```python
from build123d import *

# Parameters (mm, degrees)
BOSS_EXTRUDE2_DEPTH     = 8.3
CIRPATTERN1_COUNT       = 4
SKETCH13_R              = 22.4
CUT_EXTRUDE3_DEPTH      = 4
FILLET1_R               = 5
SKETCH15_R              = 18
SKETCH15_R_2            = 15
BOSS_EXTRUDE3_DEPTH     = 4
SKETCH16_R              = 7.5
CUT_EXTRUDE4_DEPTH      = 103.587698187
FILLET2_R               = 5
FILLET4_R               = 3
FILLET5_R               = 2
FILLET6_R               = 2
TAP_DRILL_FOR_M6_TAP1_D = 5
CIRPATTERN2_COUNT       = 4


with BuildPart() as part:
    # Sketch1 → Revolve1 (revolve)
    with BuildSketch(Plane.XY, mode=Mode.PRIVATE) as revolve1_sk:
        Polygon((22.3, -26.9), (53.8, -26.9), (53.8, 0.95810827), (56.6, 0.95810827), (56.6, 3.75810827), (59, 3.75810827), (59, 0), (59, -31.9), (0, -31.9), (0, -26.9), (17.5, -26.9), (17.5, -6.8), (22.3, -6.8), align=None)
    revolve(revolve1_sk.sketch.rotate(Axis((0, -26.9, 0), (0, -1, 0)), 180), axis=Axis((0, -26.9, 0), (0, -1, 0)))

    # Sketch2 → Boss-Extrude2 (add)
    with BuildSketch(Plane(origin=(0, 3.75810827, 0), x_dir=(1, 0, 0), z_dir=(0, 1, 0))):
        Polygon((7.756499668, 69), (-8.243500332, 69), (-11.893500332, 57.788793462), (11.406499668, 57.88688768), align=None)
    boss_extrude2 = extrude(amount=-BOSS_EXTRUDE2_DEPTH)

    # CirPattern1: Boss-Extrude2 ×4 about axis
    cirpattern1_axis = Axis((0, 0, 0), (0, 1, 0))
    for i in range(1, CIRPATTERN1_COUNT):
        add(boss_extrude2.rotate(cirpattern1_axis, i * 360 / CIRPATTERN1_COUNT))

    # Sketch10 → Cut-Revolve4 (revolve, cut)
    with BuildSketch(Plane(origin=(0, 0, 0), x_dir=(0, 0, -1), z_dir=(1, 0, 0)), mode=Mode.PRIVATE) as cut_revolve4_sk:
        Polygon((59.74122217, -25.056663082), (55.637901582, -24.521737202), (54.676040662, -31.9), (59.74122217, -32.409345916), align=None)
    revolve(cut_revolve4_sk.sketch.rotate(Axis((0, -1.306352148, 0), (0, -1, 0)), 281.147212692), axis=Axis((0, -1.306352148, 0), (0, -1, 0)), mode=Mode.SUBTRACT)

    # Sketch8 → Cut-Revolve5 (revolve, cut)
    with BuildSketch(Plane(origin=(0, 0, 0), x_dir=(0, 0, -1), z_dir=(1, 0, 0)), mode=Mode.PRIVATE) as cut_revolve5_sk:
        Polygon((57.88688768, -4.54189173), (59, -4.54189173), (59, -31.9), (56, -31.9), align=None)
    revolve(cut_revolve5_sk.sketch.rotate(Axis((0, 5.358719866, 0), (0, -1, 0)), 180), axis=Axis((0, 5.358719866, 0), (0, -1, 0)), mode=Mode.SUBTRACT)

    # Sketch12 → Cut-Revolve6 (revolve, cut)
    with BuildSketch(Plane(origin=(0, 0, 0), x_dir=(0, 0, -1), z_dir=(1, 0, 0))):
        Polygon((-55.049732908, -31.9), (-54.904154696, -30.15017811), (-17.788536772, -31.9), align=None)
    revolve(axis=Axis((0, 13.859698408, 0), (0, -1, 0)), mode=Mode.SUBTRACT)

    # Sketch13 → Cut-Extrude3 (cut)
    with BuildSketch(Plane.XZ.offset(31.9)):
        Circle(SKETCH13_R)
    extrude(amount=-CUT_EXTRUDE3_DEPTH, mode=Mode.SUBTRACT)

    # Fillet1
    # the kernel refuses this fillet: 5 mm, written as the material it takes off along each edge
    with BuildSketch(Plane(origin=(0, -31.68259181, 0), x_dir=(0, 0, 1), z_dir=(1, 0, 0))) as fillet1_piece_1:
        with BuildLine():
            CenterArc((27.185563904, -5.231169776), FILLET1_R, 87.300779723, 75.858290504)
            Line((22.4, -3.78259181), (22.304288722, -3.753620251))
            ThreePointArc((22.304288722, -3.753620251), (22.3, -1.891295905), (22.3, 0))
            Line((22.3, 0), (22.404709286, 0.099889052))
            Line((22.404709286, 0.099889052), (27.425737475, -0.136828145))
            Line((27.425737475, -0.136828145), (27.421028189, -0.236717197))
        make_face()
    revolve(axis=Axis((0, -31.68259181, 0), (0, -1, 0)), revolution_arc=270, mode=Mode.SUBTRACT)
    with BuildSketch(Plane(origin=(0, -31.68259181, 0), x_dir=(1, 0, 0), z_dir=(0, 0, -1))) as fillet1_piece_2:
        with BuildLine():
            CenterArc((27.185563904, -5.231169776), FILLET1_R, 87.300779723, 75.858290504)
            Line((22.4, -3.78259181), (22.304288722, -3.753620251))
            ThreePointArc((22.304288722, -3.753620251), (22.3, -1.891295905), (22.3, 0))
            Line((22.3, 0), (22.404709286, 0.099889052))
            Line((22.404709286, 0.099889052), (27.425737475, -0.136828145))
            Line((27.425737475, -0.136828145), (27.421028189, -0.236717197))
        make_face()
    revolve(axis=Axis((0, -31.68259181, 0), (0, -1, 0)), revolution_arc=90, mode=Mode.SUBTRACT)

    # Sketch15 → Boss-Extrude3 (add)
    with BuildSketch(Plane.XZ.offset(27.9)):
        Circle(SKETCH15_R)
        Circle(SKETCH15_R_2, mode=Mode.SUBTRACT)
    extrude(amount=BOSS_EXTRUDE3_DEPTH)

    # Sketch16 → Cut-Extrude4 (cut, through all)
    with BuildSketch(Plane.XZ.offset(27.9)):
        Circle(SKETCH16_R)
    extrude(amount=-CUT_EXTRUDE4_DEPTH, mode=Mode.SUBTRACT)

    # Fillet2
    fillet2_edges = [part.edges().sort_by_distance(p)[0] for p in [
        (-22.4, -27.9, 0),
    ]]
    fillet(fillet2_edges, radius=FILLET2_R)

    # Fillet4
    fillet4_edges = [part.edges().sort_by_distance(p)[0] for p in [
        (11.406499668, -0.39189173, -57.88688768),
        (-11.893500332, -0.39189173, -57.788793462),
        (-57.88688768, -0.39189173, -11.406499668),
        (-57.788793462, -0.39189173, 11.893500332),
        (-11.406499668, -0.39189173, 57.88688768),
        (11.893500332, -0.39189173, 57.788793462),
        (57.88688768, -0.39189173, 11.406499668),
        (57.788793462, -0.39189173, -11.893500332),
    ]]
    fillet(fillet4_edges, radius=FILLET4_R)

    # Fillet5
    fillet5_edges = [part.edges().sort_by_distance(p)[0] for p in [
        (-8.243500332, -0.39189173, -69),
        (7.756499668, -0.39189173, -69),
        (-69, -0.39189173, 8.243500332),
        (-69, -0.39189173, -7.756499668),
        (8.243500332, -0.39189173, 69),
        (-7.756499668, -0.39189173, 69),
        (69, -0.39189173, -8.243500332),
        (69, -0.39189173, 7.756499668),
    ]]
    fillet(fillet5_edges, radius=FILLET5_R)

    # Fillet6
    # the kernel refuses this fillet: 2 mm, written as the material it takes off along each edge
    with BuildSketch(Plane(origin=(0, -24.634269562, 0), x_dir=(0, 0, 1), z_dir=(-1, 0, 0))) as fillet6_piece_1:
        with BuildLine():
            CenterArc((54.622986935, 1.835886142), FILLET6_R, 300.494611252, 55.559949074)
            Line((55.637901582, 0.112532359), (55.658199875, 0.078065284))
            ThreePointArc((55.658199875, 0.078065284), (56.064338554, 0.016601804), (56.495946338, -0.039664376))
            Line((56.495946338, -0.039664376), (56.541022351, -0.00275226))
            Line((56.541022351, -0.00275226), (56.658152184, 1.695520873))
            Line((56.658152184, 1.695520873), (56.618246983, 1.698273133))
        make_face()
    revolve(axis=Axis((0, -24.634269562, 0), (0, 1, 0)), revolution_arc=258.852787308, mode=Mode.SUBTRACT)
    with BuildSketch(Plane(origin=(0, -24.634269562, 0), x_dir=(-0.9811336895007642, 0, -0.1933305028354758), z_dir=(0.1933305028354758, 0, -0.9811336895007642))) as fillet6_piece_2:
        with BuildLine():
            CenterArc((54.622986935, 1.835886142), FILLET6_R, 300.494611252, 55.559949074)
            Line((55.637901582, 0.112532359), (55.658199875, 0.078065284))
            ThreePointArc((55.658199875, 0.078065284), (56.064338554, 0.016601804), (56.495946338, -0.039664376))
            Line((56.495946338, -0.039664376), (56.541022351, -0.00275226))
            Line((56.541022351, -0.00275226), (56.658152184, 1.695520873))
            Line((56.658152184, 1.695520873), (56.618246983, 1.698273133))
        make_face()
    revolve(axis=Axis((0, -24.634269562, 0), (0, 1, 0)), revolution_arc=101.147212692, mode=Mode.SUBTRACT)

    # Tap Drill for M6 Tap1 (through all)
    with Locations(Plane(origin=(0, 3.75810827, 0), x_dir=(1, 0, 0), z_dir=(0, 1, 0))):
        with Locations((-0.243500332, 62.31716076), (62.31716076, 0.243500332), (0.243500332, -62.31716076), (-62.31716076, -0.243500332)):
            Hole(TAP_DRILL_FOR_M6_TAP1_D / 2)

    # Sketch34 → Ø2.0 (2) Diameter Hole4 (revolve, cut)
    with BuildSketch(Plane(origin=(69, 0, -5.5), x_dir=(0, 0, -1), z_dir=(0, 1, 0))):
        Polygon((0, 0), (0, 5.600860619), (1, 5), (1, 0), align=None)
    f_2_0_2_diameter_hole4 = revolve(axis=Axis((75.35, 0, -5.5), (-1, 0, 0)), mode=Mode.SUBTRACT)

    # CirPattern2: Ø2.0 (2) Diameter Hole4 ×4 about axis
    cirpattern2_axis = Axis((0, -26.9, 0), (0, 1, 0))
    for i in range(1, CIRPATTERN2_COUNT):
        add(f_2_0_2_diameter_hole4.rotate(cirpattern2_axis, i * 360 / CIRPATTERN2_COUNT), mode=Mode.SUBTRACT)


solid = part.part
```
Model file for the job. Use its own axes, mm. A direction names the side the tool comes from. Give positions to 0.01 mm unless a question says otherwise; leave off trailing zeros. Order: outer loops, then holes, each group sorted by start corner. A loop starts at its lowest first (then second) coordinate and runs counter-clockwise, first axis right, second up.
1) Mould opens along X. For faces 3 (the flat face through (63.6, -0.3, -10)), 4 (the flat face through (-63.519, -0.334, -9.557)), 5 (the cylindrical face through (0.298, -0.45, -59.877)) say: +X half, -X half, draft (parallel to the pull), parting line (faces both ways), or undercut.
2) Wall check: probe 1 along Y at (x, z) = (-65.15, 5.5); probe 2 along Z at (x, y) = (0, -29); probe 3 along Z at (x, y) = (0, -30). Give the ranges that are in metal, low to high.
3) 3-axis set-ups, long thin cutter, end or side, ignore diameter. For faces 1 (the flat face through (50, 0.958, 21)), 2 (the flat face through (9.557, -0.334, -63.519)): which of +Z, -Z, +X, -X, +Y, -Y reach the whole face in a straight line?
4) Pin check, flat tips, straight feed: pin 1 (6 mm diameter, centred on x = -0.24, z = -62.32, fed in from -Y); pin 2 (1 mm diameter, centred on x = -53.5, z = 16.5, fed in from +Y); pin 3 (10 mm diameter, centred on y = -24.5, z = -20.5, fed in from +X). Stop position of each tip, or through.
5) Saw through at A-A, the plane y = -15. Write the cut outline in (x, z).
6) Saw through at B-B, the plane x = 0. Count the separate pieces of the cut face and the enclosed holes in it, then the cut area to 3 significant figures.
Computed:
1. face 3: +X half
1. face 4: -X half
1. face 5: undercut
2. probe 1: y = -4.54 to -1, 1 to 3.76
2. probe 2: z = -55.05 to -22.67, -18 to -15, 15 to 18, 22.67 to 55.05
2. probe 3: z = -54.92 to -23.66, -18 to -15, 15 to 18, 23.66 to 54.92
3. face 1: +Y
3. face 2: -Z, +X, +Y, -Y
4. pin 1: stops at y = -4.54
4. pin 2: stops at y = 0.96
4. pin 3: stops at x = 54.38
5. outline: circle Ø114.33 at (0, 0); circle Ø44.6 at (0, 0); hole circle Ø107.6 at (0, 0); hole circle Ø35 at (0, 0)
6. separate pieces: 4
6. enclosed holes: 0
6. area: 798 mm2
